Could you check a few things on this model? Use its own coordinates, in mm. Give positions to 0.01 mm unless a question says otherwise; leave off trailing zeros. Loops run counter-clockwise (first coordinate to the right, second up) from the corner with the lowest first, then second, coordinate; pieces in that order, holes last. Notation, with made-up numbers: (-12, 72.25) -> (-8, 72.25) arc R24 cw to (-8, 91.25) -> close; hole circle Ø1 at (20, -20.75). An arc over 180 degrees is marked (long way). Write item = value, one per line. Start each with the question number.
1) I'm going to push flat-ended pins straight in: pin 1 Ø12 at (y, z) = (-13, 74.5) entering from -X; pin 2 Ø5 at (y, z) = (-22, 51) entering from -X; pin 3 Ø1 at (x, y) = (64.5, -17) entering from +Z. Where does each tip first touch, or does it pass through?
2) I want a section at D-D (x = 132.5). List the corners of the cut face in (y, z) for me, and give its area (3 significant figures).
3) I need wall thicknesses on probe 1 along X at (y, z) = (-8, 78); probe 2 along Z at (x, y) = (170, -13.25); probe 3 along X at (y, z) = (-17.5, 42). Which ranges of each line are inside material? Lowest first, please. Write a range as from..to.
4) I want a section at B-B (x = 182). List the corners of the cut face in (y, z) for me.
5) I want a section at C-C (z = -85.5). List the corners of the cut face in (x, y) for me, and give its area (3 significant figures).
6) If we mould it in two halves opening along X, with no side actions, what happens to faces 1 (the face through (36, -12, 0)), 2 (the face through (0, -12, -89)), 3 (the face through (98.49, -12.32, -116.04)), 4 (the face through (143.02, -12.32, 43.18))? For each: +X half, -X half, draft (parallel to the pull), parting line (faces both ways), or undercut.
7) I want a section at A-A (y = -20.5). List the corners of the cut face in (x, z) for me, and give its area (3 significant figures).
from build123d import *

# Parameters (mm, degrees)
F0_R     = 34
F1_DEPTH = 25
F2_DEPTH = 25


with BuildPart() as f1:
    # F0 (on Front) → F1 (new body)
    with BuildSketch(Plane.XZ):
        with BuildLine():
            Line((70.503501, 0), (0, 0))
            Line((0, 0), (0, -180))
            Line((0, -180), (199.785951, -50.254189))
            ThreePointArc((199.785951, -50.254189), (213.152795, -35.793765), (218, -16.707619))
            Line((218, -16.707619), (218, 63.868526))
            ThreePointArc((218, 63.868526), (162.994118, 16.382553), (124.045099, 77.730239))
            Line((124.045099, 77.730239), (108.716917, 28.179049))
            ThreePointArc((108.716917, 28.179049), (94.243362, 7.806538), (70.503501, 0))
        make_face()
        with BuildLine():
            ThreePointArc((218, 63.868526), (177.005882, 111.354498), (124.045099, 77.730239))
            ThreePointArc((124.045099, 77.730239), (162.994118, 16.382553), (218, 63.868526))
        make_face()
        with Locations((170, 63.868526)):
            Circle(F0_R, mode=Mode.SUBTRACT)
    extrude(amount=F1_DEPTH)

    # F0 (on Front) → F2 (join)
    with BuildSketch(Plane.XZ):
        with BuildLine():
            Line((70.503501, 0), (0, 0))
            Line((0, 0), (0, -180))
            Line((0, -180), (199.785951, -50.254189))
            ThreePointArc((199.785951, -50.254189), (213.152795, -35.793765), (218, -16.707619))
            Line((218, -16.707619), (218, 63.868526))
            ThreePointArc((218, 63.868526), (162.994118, 16.382553), (124.045099, 77.730239))
            Line((124.045099, 77.730239), (108.716917, 28.179049))
            ThreePointArc((108.716917, 28.179049), (94.243362, 7.806538), (70.503501, 0))
        make_face()
        with BuildLine():
            ThreePointArc((218, 63.868526), (177.005882, 111.354498), (124.045099, 77.730239))
            ThreePointArc((124.045099, 77.730239), (162.994118, 16.382553), (218, 63.868526))
        make_face()
        with Locations((170, 63.868526)):
            Circle(F0_R, mode=Mode.SUBTRACT)
    extrude(amount=F2_DEPTH)


solid = f1.part
Answer list:
q1.pin_1 = 121.19
q1.pin_2 = 115
q1.pin_3 = 0
q2.outline = (-25, -93.95) -> (0, -93.95) -> (0, 93.83) -> (-25, 93.83) -> close
q2.area = 4,690 mm^2
q3.probe_1 = 124.13..139.08, 200.92..215.87
q3.probe_2 = -69.6..29.87, 97.87..111.87
q3.probe_3 = 112.99..143.97, 196.03..218
q4.outline = (-25, -61.8) -> (0, -61.8) -> (0, 32.06) -> (-25, 32.06) -> close; (-25, 95.68) -> (0, 95.68) -> (0, 110.34) -> (-25, 110.34) -> close
q5.outline = (0, -25) -> (145.51, -25) -> (145.51, 0) -> (0, 0) -> close
q5.area = 3,640 mm^2
q6.face_1 = draft
q6.face_2 = -X half
q6.face_3 = +X half
q6.face_4 = undercut
q7.outline = (0, -180) -> (199.79, -50.25) arc R40 ccw to (218, -16.71) -> (218, 63.87) arc R48 ccw to (124.05, 77.73) -> (108.72, 28.18) arc R40 cw to (70.5, 0) -> (0, 0) -> close; hole circle Ø68 at (170, 63.87)
q7.area = 30,800 mm^2
